The figure shows three views and two pictorial views of one solid part (mm, origin at its lowest corner). Answer the questions. Give positions to 0.01 mm unless a question says otherwise; leave off trailing zeros. Loops run counter-clockwise (first coordinate to the right, second up) from the corner with the lowest first, then second, coordinate; pieces in that order, holes last. Notation, with made-up numbers: M -40,-14 L -11,-14 A32 cw -11,13 Z; hole C -14.75,-5 d10. An arc over 180 degrees is marked long. Answer as a JSON object with one key per item and string values. Group by question number.
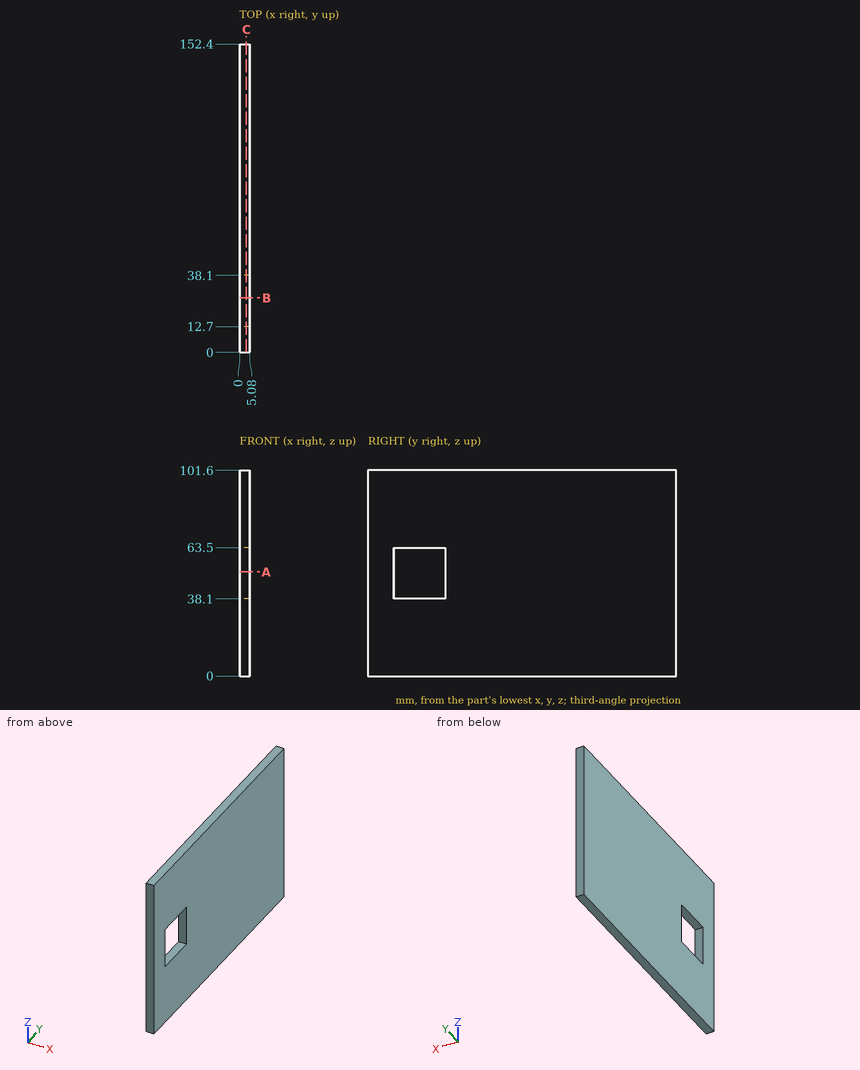
Item 1: A cutting plane is placed at B-B (y = 27). Determine the outline of the cut face in (x, z).
Item 2: Find the intervals of material crossed by probe 1 along Z at (x, y) = (4.5, 16); probe 2 along Y at (x, z) = (1.75, 57.5), in increasing order. Write a range as [from, to].
Item 3: A cutting plane is placed at A-A (z = 51.5). Determine the outline of the cut face in (x, y), and give its area (3 significant figures).
Item 4: A cutting plane is placed at C-C (x = 3.35). Determine the outline of the cut face in (y, z).
The answers:
{
 "1": {"outline": "M 0,0 L 5.08,0 L 5.08,38.1 L 0,38.1 Z; M 0,63.5 L 5.08,63.5 L 5.08,101.6 L 0,101.6 Z"},
 "2": {"probe 1": "z = [0, 38.1], [63.5, 101.6]", "probe 2": "y = [0, 12.7], [38.1, 152.4]"},
 "3": {"outline": "M 0,0 L 5.08,0 L 5.08,12.7 L 0,12.7 Z; M 0,38.1 L 5.08,38.1 L 5.08,152.4 L 0,152.4 Z", "area": "645 mm^2"},
 "4": {"outline": "M 0,0 L 152.4,0 L 152.4,101.6 L 0,101.6 Z; hole M 12.7,38.1 L 38.1,38.1 L 38.1,63.5 L 12.7,63.5 Z"}
}
